```python
from build123d import *

# Parameters (mm, degrees)
SKETCH1_W           = 94
SKETCH1_H           = 63
BOSS_EXTRUDE1_DEPTH = 31
FILLET1_R           = 6.35
SKETCH3_W           = 50.5
SKETCH3_H           = 2
BOSS_EXTRUDE2_DEPTH = 2.5
SKETCH4_W           = 8.5
SKETCH4_H           = 3.8
CUT_EXTRUDE1_DEPTH  = 8
SKETCH5_R           = 8.5
SKETCH5_R_2         = 3.5
SKETCH5_W           = 3.5
SKETCH5_H           = 3.5
CUT_EXTRUDE2_DEPTH  = 2
SKETCH6_R           = 1.5875
CUT_EXTRUDE3_DEPTH  = 5


with BuildPart() as part:
    # Sketch1 → Boss-Extrude1 (new body)
    with BuildSketch(Plane(origin=(0, 0, 0), x_dir=(1, 0, 0), z_dir=(0, 1, 0))):
        with Locations((47, 31.5)):
            Rectangle(SKETCH1_W, SKETCH1_H)
    extrude(amount=BOSS_EXTRUDE1_DEPTH)

    # Fillet1
    fillet1_edges = [part.edges().sort_by_distance(p)[0] for p in [
        (0, 15.5, 0),
        (0, 15.5, -63),
        (94, 15.5, -63),
        (94, 15.5, 0),
    ]]
    fillet(fillet1_edges, radius=FILLET1_R)

    # Sketch3 → Boss-Extrude2 (add)
    with BuildSketch(Plane(origin=(0, 0, -63), x_dir=(-1, 0, 0), z_dir=(0, 0, -1))):
        with Locations((-37.25, 27.46)):
            Rectangle(SKETCH3_W, SKETCH3_H)
    extrude(amount=BOSS_EXTRUDE2_DEPTH)

    # Sketch4 → Cut-Extrude1 (cut)
    with BuildSketch(Plane.XY):
        with Locations((14.45, 9.65)):
            Rectangle(SKETCH4_W, SKETCH4_H)
    extrude(amount=-CUT_EXTRUDE1_DEPTH, mode=Mode.SUBTRACT)

    # Sketch5 → Cut-Extrude2 (cut)
    with BuildSketch(Plane(origin=(0, 31, 0), x_dir=(1, 0, 0), z_dir=(0, 1, 0))):
        with Locations((47, 31.5)):
            Circle(SKETCH5_R)
        with Locations((53.01040764, 37.51040764)):
            Circle(SKETCH5_R_2)
        with Locations((53.01040764, 25.48959236)):
            Circle(SKETCH5_R_2)
        with Locations((54.76040764, 39.26040764)):
            Rectangle(SKETCH5_W, SKETCH5_H)
        with Locations((54.76040764, 23.73959236)):
            Rectangle(SKETCH5_W, SKETCH5_H)
    extrude(amount=-CUT_EXTRUDE2_DEPTH, mode=Mode.SUBTRACT)

    # Sketch6 → Cut-Extrude3 (cut)
    with BuildSketch(Plane.XZ):
        with Locations((27.2, -31.5)):
            Circle(SKETCH6_R)
        with Locations((79, -31.5)):
            Circle(SKETCH6_R)
    extrude(amount=-CUT_EXTRUDE3_DEPTH, mode=Mode.SUBTRACT)


solid = part.part
```
Could you check a few things on this model? Use its own coordinates, in mm. A direction names the side the tool comes from. Coordinates: 2 decimals unless noted, no trailing zeros. Loops run counter-clockwise (first coordinate to the right, second up) from the corner with the lowest first, then second, coordinate; pieces in that order, holes last. Notation, with made-up numbers: M 7,-4 L 47,-4 A25 ccw 47,9 Z; hole C -6,66.25 d6. An arc over 180 degrees is marked long. Put each result on its own line as item: value. Start each with the question number.
(1) Suppose I cut it at B-B on y = 2. Count the separate pieces of the cut face and the enclosed holes in it, then the cut area to 3 significant figures.
(2) Suppose I cut it at A-A on x = 47. Please give me the cut outline in (y, z), then the cut area to 3 significant figures.
(3) For faces 1 (the face through (1.81, 15.72, -61.09)), 2 (the face through (14, 7.75, -4)), 3 (the face through (55, 30, -21.99)), 4 (the face through (25.614, 2.465, -31.43)), which set-ups out of +Z, -Z, +X, -X, +Y, -Y let a thin tool reach every point of the face, with its end or its side?
(4) Suppose I cut it at D-D on y = 24. Please give me the cut outline in (x, z).
(5) I need wall thicknesses on line 1 (Z direction, x = 27.2, y = 2.9); line 2 (X direction, y = 30, z = -31); line 3 (Z direction, x = 80, y = 23). Which ranges of each line are inside material? Lowest first, please. Write a range as from..to.
(6) Suppose I cut it at C-C on z = -31.5. Please give me the cut outline in (x, y), then the cut area to 3 significant figures.
(7) Thinking about a two-plate mould opening in Y: for faces 5 (the face through (38, 26.46, -64)), 6 (the face through (55.5, 30, -31.5)), 7 (the face through (18.7, 10, -4)), 8 (the face through (38, 28.46, -64)), which applies, pulls with the +Y half, pulls with the -Y half, needs draft (parallel to the pull), parting line crosses it, or undercut?
(8) Will these pins go through, and if not, where does the flat tip stop? P1, Ø2.5, axis at x = 79, z = -31, coming from the -Y side; P2, Ø2, axis at x = 47.5, z = -64.5, coming from the -Y side; P3, Ø1.9, axis at x = 13.5, y = 9.5, coming from the +Z side; P4, Ø5.5, axis at x = 44, z = -30.5, coming from the +Y side.
Solutions:
1. separate pieces: 1
1. enclosed holes: 2
1. area: 5,870 mm2
2. outline: M 0,-63 L 26.46,-63 L 26.46,-65.5 L 28.46,-65.5 L 28.46,-63 L 31,-63 L 31,-40 L 29,-40 L 29,-23 L 31,-23 L 31,0 L 0,0 Z
2. area: 1,920 mm2
3. face 1: -Z, -X, +Y, -Y
3. face 2: +Z
3. face 3: +Y
3. face 4: -Y
4. outline: M 0,-56.65 A6.35 ccw 6.35,-63 L 87.65,-63 A6.35 ccw 94,-56.65 L 94,-6.35 A6.35 ccw 87.65,0 L 6.35,0 A6.35 ccw 0,-6.35 Z
5. line 1: z = -63..-33.09, -29.91..0
5. line 2: x = 0..38.51, 55.49..94
5. line 3: z = -63..0
6. outline: M 0,0 L 25.61,0 L 25.61,5 L 28.79,5 L 28.79,0 L 77.41,0 L 77.41,5 L 80.59,5 L 80.59,0 L 94,0 L 94,31 L 55.5,31 L 55.5,29 L 38.5,29 L 38.5,31 L 0,31 Z
6. area: 2,850 mm2
7. face 5: pulls with the -Y half
7. face 6: needs draft
7. face 7: undercut
7. face 8: pulls with the +Y half
8. P1: stops at y = 0
8. P2: stops at y = 26.46
8. P3: stops at z = -8
8. P4: stops at y = 29
